Verification items for the finished model (mm, model axes). A direction names the side the tool comes from. Coordinates: 2 decimals unless noted, no trailing zeros. Order: outer loops, then holes, each group sorted by start corner. A loop starts at its lowest first (then second) coordinate and runs counter-clockwise, first axis right, second up.
Q1. Cross-section at D-D, the plane y = -4.75. Record the boundary of the cut face in (x, z), and give its area (3 significant figures).
Q2. Draft check along Y on faces 5 (the flat face through (11.68, 2.96, -7.44)), 6 (the cylindrical face through (-15.77, 2.43, -17.73)), 7 (the conical face through (-0.073, 1.775, 9.903)). Enter one of: pulls with the +Y half, pulls with the -Y half, needs draft (parallel to the pull), parting line crosses it, or undercut.
Q3. Thickness scan on line 1 (Y direction, x = 0, z = 13.75); line 2 (X direction, y = -4, z = 0); line 3 (X direction, y = -5.95, z = 0). Record the ranges inside material, lowest first.
Q4. Cross-section at B-B, the plane x = 0. Count the separate pieces of the cut face and the enclosed holes in it, and give its area (3 significant figures).
Q5. Set-up check for faces 1 (the cylindrical face through (-17.73, 2.43, 15.77)), 2 (the flat face through (15, -3, 23)), 3 (the flat face through (11, 0, 11)), 4 (the cylindrical face through (8.178, 4.732, 0.047)): record each of +Z, -Z, +X, -X, +Y, -Y from which the full face is reachable in a straight line by a thin tool's end or side.
Q6. Cross-section at C-C, the plane y = 5.25. Record the boundary of the cut face in (x, z), and give its area (3 significant figures).
Q7. Depth check by flat-ended pin: P1, Ø2, axis at y = 1, z = -13, coming from the +X side; P2, Ø13, axis at x = 3, z = 9, coming from the -Y side; P3, Ø4, axis at y = 4, z = 16, coming from the -X side; P4, Ø5, axis at x = 9, z = 9, coming from the +Y side. Enter the tip coordinate at first touch or a pass-through.
from build123d import *

# Parameters (mm, degrees)
SKETCH1_R               = 27.889608224
BOSS_EXTRUDE1_DEPTH     = 6
CUT_EXTRUDE1_REACH      = 61.354
CUT_EXTRUDE1_END_RADIUS = 27.889608224
SKETCH2_R               = 1.5
CIRPATTERN1_COUNT       = 4
CHAMFER1_SIZE           = 3.5
BOSS_EXTRUDE2_START     = 6
SKETCH3_R               = 27.889608224
SKETCH3_R_2             = 11.678118969
BOSS_EXTRUDE2_DEPTH     = 6
CUT_EXTRUDE2_REACH      = 64.651
SKETCH4_R               = 1
SKETCH5_R               = 27.889608224
SKETCH5_R_2             = 26.889608224
SKETCH5_R_3             = 25.031826588
SKETCH5_R_4             = 19.031826588
CUT_EXTRUDE3_DEPTH      = 3
FILLET1_R               = 3


with BuildPart() as part:
    # Sketch1 → Boss-Extrude1 (new body)
    with BuildSketch(Plane(origin=(0, 0, 0), x_dir=(1, 0, 0), z_dir=(0, 1, 0))):
        with Locations(Location((0, 0, 0), (0, 0, 270))):
            Circle(SKETCH1_R)
        with BuildLine():
            ThreePointArc((-7.500987149, 3.258346461), (-8.178118969, 0), (-7.500987149, -3.258346461))
            Line((-7.500987149, -3.258346461), (-15.986268523, -11.743627836))
            Line((-15.986268523, -11.743627836), (-11.743627836, -15.986268523))
            Line((-11.743627836, -15.986268523), (-3.258346461, -7.500987149))
            ThreePointArc((-3.258346461, -7.500987149), (0, -8.178118969), (3.258346461, -7.500987149))
            Line((3.258346461, -7.500987149), (11.743627836, -15.986268523))
            Line((11.743627836, -15.986268523), (15.986268523, -11.743627836))
            Line((15.986268523, -11.743627836), (7.500987149, -3.258346461))
            ThreePointArc((7.500987149, -3.258346461), (8.178118969, 0), (7.500987149, 3.258346461))
            Line((7.500987149, 3.258346461), (15.986268523, 11.743627836))
            Line((15.986268523, 11.743627836), (11.743627836, 15.986268523))
            Line((11.743627836, 15.986268523), (3.258346461, 7.500987149))
            ThreePointArc((3.258346461, 7.500987149), (0, 8.178118969), (-3.258346461, 7.500987149))
            Line((-3.258346461, 7.500987149), (-11.743627836, 15.986268523))
            Line((-11.743627836, 15.986268523), (-15.986268523, 11.743627836))
            Line((-15.986268523, 11.743627836), (-7.500987149, 3.258346461))
        make_face(mode=Mode.SUBTRACT)
    extrude(amount=BOSS_EXTRUDE1_DEPTH)

    # Cut-Extrude1: up to this cylinder (the profile starts inside it)
    cut_extrude1_end = Plane(origin=(0, 3, 0), z_dir=(0, -1, 0)) * Cylinder(CUT_EXTRUDE1_END_RADIUS, 179.487216449, mode=Mode.PRIVATE)
    # Sketch2 → Cut-Extrude1 (cut, up to the surface)
    with BuildSketch(Plane(origin=(13.864948179, 0, -13.864948179), x_dir=(0.7071067811865458, 0, 0.7071067811865492), z_dir=(-0.7071067811865492, 0, 0.7071067811865458)), mode=Mode.PRIVATE) as cut_extrude1_sk1:
        with Locations((0, 3)):
            Circle(SKETCH2_R)
    cut_extrude1_tool1 = extrude(cut_extrude1_sk1.sketch, amount=-CUT_EXTRUDE1_REACH, mode=Mode.PRIVATE) & cut_extrude1_end
    cut_extrude1 = cut_extrude1_tool1.solids().sort_by_distance((13.864948, 3, -13.864948))[0]
    add(cut_extrude1, mode=Mode.SUBTRACT)

    # CirPattern1: Cut-Extrude1 ×4 about axis
    cirpattern1_axis = Axis((0, 6, 0), (0, -1, 0))
    for i in range(1, CIRPATTERN1_COUNT):
        add(cut_extrude1.rotate(cirpattern1_axis, i * 360 / CIRPATTERN1_COUNT), mode=Mode.SUBTRACT)

    # Chamfer1
    chamfer1_edges = [part.edges().sort_by_distance(p)[0] for p in [
        (0, 0, 8.178118969),
        (8.178118969, 0, 0),
        (0, 0, -8.178118969),
        (-8.178118969, 0, 0),
    ]]
    chamfer(chamfer1_edges, length=CHAMFER1_SIZE)

    # Sketch3 → Boss-Extrude2 (add)
    with BuildSketch(Plane.XZ.offset(BOSS_EXTRUDE2_START)):
        with Locations(Location((0, 0, 0), (0, 0, 270))):
            Circle(SKETCH3_R)
        with Locations(Location((0, 0, 0), (0, 0, 59.885646145))):
            Circle(SKETCH3_R_2, mode=Mode.SUBTRACT)
    extrude(amount=-BOSS_EXTRUDE2_DEPTH)

    # Sketch4 → Cut-Extrude2 (cut, up to next)
    with BuildSketch(Plane.XY.offset(27.889608224), mode=Mode.PRIVATE) as cut_extrude2_sk1:
        with Locations((0, 3.461741733)):
            Circle(SKETCH4_R)
    cut_extrude2_tool1 = extrude(cut_extrude2_sk1.sketch, amount=-CUT_EXTRUDE2_REACH, mode=Mode.PRIVATE) & part.part
    add(cut_extrude2_tool1.solids().sort_by_distance((0, 3.461742, 27.889608))[0], mode=Mode.SUBTRACT)

    # Sketch5 → Cut-Extrude3 (cut)
    # profile 1 of 2: a face of its own
    with BuildSketch(Plane.XZ.offset(6)):
        with Locations(Location((0, 0, 0), (0, 0, 270))):
            Circle(SKETCH5_R)
        with Locations(Location((0, 0, 0), (0, 0, 270))):
            Circle(SKETCH5_R_2, mode=Mode.SUBTRACT)
    # profile 2 of 2: a face of its own
    with BuildSketch(Plane.XZ.offset(6)):
        with Locations(Location((0, 0, 0), (0, 0, 270))):
            Circle(SKETCH5_R_3)
        with Locations(Location((0, 0, 0), (0, 0, 270))):
            Circle(SKETCH5_R_4, mode=Mode.SUBTRACT)
    extrude(amount=-CUT_EXTRUDE3_DEPTH, mode=Mode.SUBTRACT)

    # Fillet1
    fillet1_edges = [part.edges().sort_by_distance(p)[0] for p in [
        (0, -3, 25.031826588),
        (0, -3, 19.031826588),
    ]]
    fillet(fillet1_edges, radius=FILLET1_R - 0.0001)  # a hair under: the kernel refuses the full size


solid = part.part
Check values:
1. outline: circle Ø53.78 at (0, 0); circle Ø38.61 at (0, 0); hole circle Ø49.52 at (0, 0); hole circle Ø23.36 at (0, 0)
1. area: 1,090 mm2
2. face 5: needs draft
2. face 6: undercut
2. face 7: pulls with the -Y half
3. line 1: y = -6 to 2.46, 4.46 to 6
3. line 2: x = -26.89 to -24.27, -19.8 to -11.68, 11.68 to 19.8, 24.27 to 26.89
3. line 3: x = -26.89 to -25.03, -19.03 to -11.68, 11.68 to 19.03, 25.03 to 26.89
4. separate pieces: 3
4. enclosed holes: 0
4. area: 346 mm2
5. face 1: none
5. face 2: -Y
5. face 3: +Y
5. face 4: +Y, -Y
6. outline: circle Ø55.78 at (0, 0); hole (-15.99, -11.74) - (-11.74, -15.99) - (-3.26, -7.5) arc R8.18 ccw to (3.26, -7.5) - (11.74, -15.99) - (15.99, -11.74) - (7.5, -3.26) arc R8.18 ccw to (7.5, 3.26) - (15.99, 11.74) - (11.74, 15.99) - (3.26, 7.5) arc R8.18 ccw to (-3.26, 7.5) - (-11.74, 15.99) - (-15.99, 11.74) - (-7.5, 3.26) arc R8.18 ccw to (-7.5, -3.26) - close
6. area: 1,950 mm2
7. P1: stops at x = 25.18
7. P2: stops at y = -6
7. P3: stops at x = -24.12
7. P4: stops at y = 0
